Part model, mm, in its own coordinate system. Face numbers are marked on the shaded views. Coordinates: 2 decimals unless noted, no trailing zeros. Write each loop counter-clockwise with the first axis right and the second up, starting at its lowest first coordinate (ties: lowest second). Pieces come first, ordered by that corner, then holes. Notation, with made-up numbers: (-29.75, 82) - (26.25, 82) arc R31 cw to (26.25, 113) - close; hole circle Ø6 at (31, 47). An arc over 180 degrees is marked (long way). Use a Markdown table: item, result.
```python
from build123d import *

# Parameters (mm, degrees)
BOSS_EXTRUDE1_DEPTH     = 338.4
CUT_EXTRUDE1_DEPTH      = 4078.516360054
BODY_MOVE_COPY1_ANGLE   = 6.4948363
CUT_EXTRUDE2_DEPTH      = 1007.656101098
CUT_EXTRUDE2_DEPTH_BACK = 1007.656101098
SKETCH8_R               = 25


with BuildPart() as part:
    # Sketch1 → Boss-Extrude1 (new body)
    with BuildSketch(Plane(origin=(-169.199995481, 0.039105561, 0), x_dir=(-0.00023112033831648726, -0.9999999732916943, 0), z_dir=(-0.9999999732916943, 0.00023112033831648726, -9.983680815562587e-14))):
        with BuildLine():
            Line((-8457.49603755, 2990.648405965), (-8376.54968012, 2279.62014296))
            ThreePointArc((-8376.54968012, 2279.62014296), (-8237.524375906, 2169.013910965), (-8126.918143911, 2308.039215179))
            Line((-8126.918143911, 2308.039215179), (-8207.864501341, 3019.067478184))
            ThreePointArc((-8207.864501341, 3019.067478184), (-8346.889805555, 3129.673710179), (-8457.49603755, 2990.648405965))
        make_face()
    extrude(amount=-BOSS_EXTRUDE1_DEPTH)

    # Sketch2 → Cut-Extrude1 (cut, through all)
    with BuildSketch(Plane(origin=(1.794312536, 7763.54214826, -883.833325812), x_dir=(0.9999999736334177, -0.00022816323452923984, 2.597503388930373e-05), z_dir=(-0.0002296370265797643, -0.9935820538684025, 0.11311343641443838))):
        Polygon((60.107789667, 4123.109536872), (-59.892210195, 4123.11267401), (-59.900592157, 3802.490672498), (60.099407705, 3802.48753536), align=None)
    extrude(amount=-CUT_EXTRUDE1_DEPTH, mode=Mode.SUBTRACT)

    # Sketch3 → Revolve1 (revolve)
    with BuildSketch(Plane(origin=(2e-09, 0, 3004.857942074), x_dir=(-1, 0, 0), z_dir=(0, 0, -1)), mode=Mode.PRIVATE) as revolve1_sk:
        Polygon((-61.943184257, 8407.666177671), (-61.925850231, 8332.666179674), (58.07414647, 8332.693914114), (58.056812444, 8407.693912112), align=None)
    revolve(revolve1_sk.sketch.rotate(Axis((61.925850233, 8332.666179674, 3004.857942074), (-0.9999999732916957, 0.0002311203324015103, 5.403085390737201e-13)), 180), axis=Axis((61.925850233, 8332.666179674, 3004.857942074), (-0.9999999732916957, 0.0002311203324015103, 5.403085390737201e-13)))

    # Sketch4 → Revolve2 (revolve)
    with BuildSketch(Plane(origin=(1e-09, 0, 2293.82967907), x_dir=(-1, 0, 0), z_dir=(0, 0, -1)), mode=Mode.PRIVATE) as revolve2_sk:
        Polygon((-371.124467697, 8326.648359994), (-371.107133671, 8251.648361997), (-171.107139013, 8251.694586065), (-171.124473038, 8326.694584062), align=None)
    revolve(revolve2_sk.sketch.rotate(Axis((371.107122989, 8251.648361999, 2293.829679069), (-0.9999999732916943, 0.0002311203383076049, 5.395684476116649e-13)), 180), axis=Axis((371.107122989, 8251.648361999, 2293.829679069), (-0.9999999732916943, 0.0002311203383076049, 5.395684476116649e-13)))

    # Sketch5 → Revolve3 (revolve)
    with BuildSketch(Plane(origin=(2e-09, 0, 3004.857942074), x_dir=(-1, 0, 0), z_dir=(0, 0, -1)), mode=Mode.PRIVATE) as revolve3_sk:
        Polygon((-371.143176046, 8407.594715262), (-371.12584202, 8332.594717265), (-171.125847362, 8332.640941332), (-171.143181387, 8407.640939329), align=None)
    revolve(revolve3_sk.sketch.rotate(Axis((371.125831339, 8332.594717267, 3004.857942074), (-0.9999999732916943, 0.00023112033830760464, 5.395684476116643e-13)), 180), axis=Axis((371.125831339, 8332.594717267, 3004.857942074), (-0.9999999732916943, 0.00023112033830760464, 5.395684476116643e-13)))

    # Sketch6 → Revolve4 (revolve)
    with BuildSketch(Plane(origin=(1e-09, 0, 2293.82967907), x_dir=(-1, 0, 0), z_dir=(0, 0, -1)), mode=Mode.PRIVATE) as revolve4_sk:
        Polygon((167.275517924, 8326.772795184), (167.292851949, 8251.772797187), (367.292846607, 8251.819021255), (367.275512582, 8326.819019252), align=None)
    revolve(revolve4_sk.sketch.rotate(Axis((-167.292862631, 8251.77279719, 2293.82967907), (-0.9999999732916943, 0.00023112033831648596, 5.41788893898131e-13)), 180), axis=Axis((-167.292862631, 8251.77279719, 2293.82967907), (-0.9999999732916943, 0.00023112033831648596, 5.41788893898131e-13)))

    # Sketch7 → Revolve5 (revolve)
    with BuildSketch(Plane(origin=(2e-09, 0, 3004.857942074), x_dir=(-1, 0, 0), z_dir=(0, 0, -1)), mode=Mode.PRIVATE) as revolve5_sk:
        Polygon((167.256809575, 8407.719150452), (167.2741436, 8332.719152455), (367.274138258, 8332.765376523), (367.256804233, 8407.765374519), align=None)
    revolve(revolve5_sk.sketch.rotate(Axis((-167.274154282, 8332.719152457, 3004.857942075), (-0.9999999732916943, 0.00023112033831648528, 5.417888938981294e-13)), 180), axis=Axis((-167.274154282, 8332.719152457, 3004.857942075), (-0.9999999732916943, 0.00023112033831648528, 5.417888938981294e-13)))


with BuildPart() as part_1:
    # Body-Move/Copy1: read off the stored shape, not the designer's step
    # Body-Move/Copy1: moved
    add(part.part.moved(Location((1.8963, 208.8730906, -934.0697721))).rotate(Axis((0, 0, 0), (0.9999979393, 0, 0.0020301439)), BODY_MOVE_COPY1_ANGLE))


with BuildPart() as part_2:
    # Body-Move/Copy2: read off the stored shape, not the designer's step
    # Body-Move/Copy2: moved
    add(part_1.part.moved(Location((-0.0396508, -8252.5008213, -3023.6625196))))

    # Sketch8 → Cut-Extrude2 (cut, two sides: drawn at the far end of the back side and taken through both)
    with BuildSketch(Plane(origin=(171.048025075, 0, -0.002243036), x_dir=(-1.311348857824843e-05, 0, -0.9999999999140183), z_dir=(0.9999999999140183, 0, -1.311348857824843e-05)).offset(-CUT_EXTRUDE2_DEPTH_BACK)):
        with Locations(Location((158.041542403, 0, 0), (0, 0, 180))):
            Circle(SKETCH8_R)
    extrude(amount=CUT_EXTRUDE2_DEPTH + CUT_EXTRUDE2_DEPTH_BACK, mode=Mode.SUBTRACT)


solid = part_2.part
```
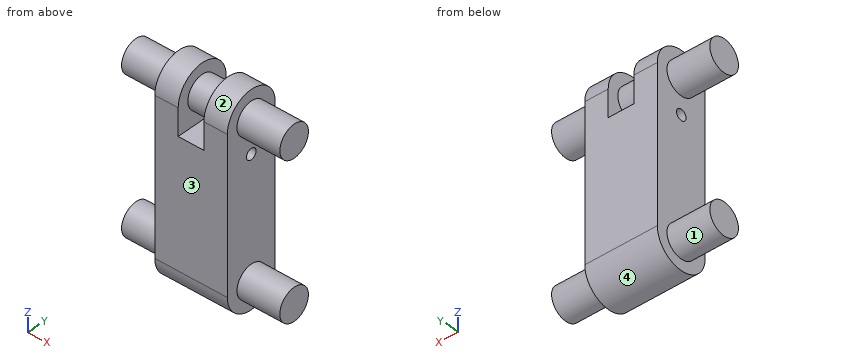
Item 1: Band-saw the part on A-A, the plane y = 0. Count the separate pieces of the cut face and the enclosed holes in it, then the cut area to 3 significant figures.
From the geometry:
| item | result |
|---|---|
| separate pieces | 2 |
| enclosed holes | 1 |
| area | 418,000 mm^2 |
Item 2: Drill centre lines: probe 1 along Z at (x, y) = (-170.5, -3.5); probe 2 along X at (y, z) = (-92, -771); probe 3 along Y at (x, z) = (-75.5, -723). Where is each one in solid material? Low to high.
From the geometry:
| item | result |
|---|---|
| probe 1 | -790.54 to -640.7, -74.92 to 74.92 |
| probe 2 | -167.36 to 171.04 |
| probe 3 | -125.41 to 125.41 |
Item 3: Two-plate mould, pull along Z, no slides. Class the marked faces 1, 2, 3 and 4: pulls with the +Z half, pulls with the -Z half, needs draft (parallel to the pull), parting line crosses it, or undercut.
From the geometry:
| item | result |
|---|---|
| face 1 | undercut |
| face 2 | pulls with the +Z half |
| face 3 | needs draft |
| face 4 | pulls with the -Z half |
Item 4: Drop flat-ended pins along their axis: P1, Ø5, axis at x = -49.5, y = -35.5, coming from the +Z side; P2, Ø1, axis at y = -30, z = -490.5, coming from the +X side; P3, Ø5, axis at x = 285, y = -1, coming from the -Z side. Give the stop position or say it passes through.
From the geometry:
| item | result |
|---|---|
| P1 | z = 67.35 |
| P2 | x = 171.04 |
| P3 | z = -790.62 |
Item 5: Band-saw the part on D-D, the plane z = -597. Give the cut face in (x, y), then the cut area to 3 significant figures.
From the geometry:
| item | result |
|---|---|
| outline | (-167.36, -125.62) - (171.04, -125.62) - (171.04, 125.62) - (-167.36, 125.62) - close |
| area | 85,000 mm^2 |
Item 6: Band-saw the part on C-C, the plane y = 96. Give the cut face in (x, z), then the cut area to 3 significant figures.
From the geometry:
| item | result |
|---|---|
| outline | (-167.36, -796.64) - (171.04, -796.65) - (171.05, 81.02) - (61.85, 81.02) - (61.85, -125.62) - (-58.15, -125.62) - (-58.15, 81.02) - (-167.35, 81.03) - close |
| area | 272,000 mm^2 |
Item 7: Band-saw the part on B-B, the plane y = 49. Give the cut face in (x, z).
From the geometry:
| item | result |
|---|---|
| outline | (-367.36, -772.4) - (-167.36, -772.4) - (-167.36, -831.29) - (171.04, -831.29) - (171.04, -772.4) - (371.04, -772.41) - (371.04, -658.85) - (171.04, -658.84) - (171.05, -56.78) - (371.05, -56.79) - (371.05, 56.78) - (171.05, 56.78) - (171.05, 115.67) - (61.85, 115.67) - (61.85, 56.78) - (-58.15, 56.78) - (-58.15, 115.67) - (-167.35, 115.67) - (-167.35, 56.78) - (-367.35, 56.79) - (-367.35, -56.78) - (-167.35, -56.78) - (-167.36, -658.84) - (-367.36, -658.84) - close; hole (-58.15, -125.62) - (61.85, -125.62) - (61.85, -56.78) - (-58.15, -56.78) - close |
